```python
from build123d import *

# Parameters (mm, degrees)
BOSS_EXTRUDE1_DEPTH = 2
CUT_EXTRUDE2_DEPTH  = 330


with BuildPart() as part:
    # Sketch1 → Boss-Extrude1 (new body)
    with BuildSketch(Plane.XY):
        Polygon((1242, 1506), (0, 1506), (0, 0), (1239.998813056, 0), (1239.998813056, -14), (1672.998813056, -14), (1672.998813056, -313), (2035, -313), (2035, 1817), (1242, 1817), align=None)
    extrude(amount=BOSS_EXTRUDE1_DEPTH)

    # Sketch3 → Cut-Extrude2 (cut)
    with BuildSketch(Plane(origin=(-124.112118138, -344, 1006.457487155), x_dir=(-1, 0, 0), z_dir=(0, -1, 0))):
        with BuildLine():
            Line((-1887.112118138, 819.457487155), (-1466.112118138, 819.457487155))
            ThreePointArc((-1466.112118138, 819.457487155), (-1395.40144002, 848.746809036), (-1366.112118138, 919.457487155))
            Line((-1366.112118138, 919.457487155), (-1366.112118138, 2569.457487155))
            ThreePointArc((-1366.112118138, 2569.457487155), (-1395.40144002, 2640.168165273), (-1466.112118138, 2669.457487155))
            Line((-1466.112118138, 2669.457487155), (-1887.112118138, 2669.457487155))
            ThreePointArc((-1887.112118138, 2669.457487155), (-1957.822796257, 2640.168165273), (-1987.112118138, 2569.457487155))
            Line((-1987.112118138, 2569.457487155), (-1987.112118138, 919.457487155))
            ThreePointArc((-1987.112118138, 919.457487155), (-1957.822796257, 848.746809036), (-1887.112118138, 819.457487155))
        make_face()
    extrude(amount=-CUT_EXTRUDE2_DEPTH, mode=Mode.SUBTRACT)


solid = part.part
```
Build history of the part. All positions in model axes, mm. Give positions to 0.01 mm unless a question says otherwise; leave off trailing zeros. Order: outer loops, then holes, each group sorted by start corner. A loop starts at its lowest first (then second) coordinate and runs counter-clockwise, first axis right, second up. Notation, with made-up numbers: M 2,-15 L 22,-15 A24 ccw 22,-5 Z; hole C 31,74 d9. An arc over 180 degrees is marked long. Write item = value, one per line. Start each with the question number.
(1) Slice it at C-C on x = 1128. Write the cut outline in (y, z), plus the area to 3 significant figures.
(2) Pin check, flat tips, straight feed: pin 1 Ø0.6 at (x, z) = (635.5, 1) entering from +Y; pin 2 Ø0.6 at (x, z) = (874, 1.5) entering from -Y; pin 3 Ø1 at (x, z) = (1418, 1) entering from -Y. Stop position of each tip, or through.
(3) Slice it at A-A on z = 1.5. Write the cut outline in (x, y).
(4) Slice it at B-B on x = 1448. Write the cut outline in (y, z), plus the area to 3 significant figures.
(5) Probe L1, parallel to Y at x = 1593.5, z = 0.15; L2, parallel to Y at x = 563.5, z = 0.3; L3, parallel to X at y = 1694, z = 0.15. List the from-to ranges inside material, lowest first. Write a range as [from, to].
Responses:
q1.outline = M 0,0 L 1506,0 L 1506,2 L 0,2 Z
q1.area = 3,010 mm2
q2.pin_1 = 1506
q2.pin_2 = 0
q2.pin_3 = -14
q3.outline = M 0,0 L 1240,0 L 1240,-14 L 1863,-14 L 1863,-313 L 2035,-313 L 2035,1817 L 1242,1817 L 1242,1506 L 0,1506 Z
q4.outline = M -14,0 L 1817,0 L 1817,2 L -14,2 Z
q4.area = 3,660 mm2
q5.L1 = [-14, 1817]
q5.L2 = [0, 1506]
q5.L3 = [1242, 2035]
